Autodesk Inventor part; units mm, degrees
ref_plane "YZ Plane" through (0, 0, 0) normal (1, 0, 0) x (0, 1, 0)
ref_plane "XZ Plane" through (0, 0, 0) normal (0, 1, 0) x (-1, 0, 0)
ref_plane "XY Plane" through (0, 0, 0) normal (0, 0, 1) x (1, 0, 0)
sketch "Sketch1" plane through (0, 0, 0) normal (0, 0, 1) x (1, 0, 0)
  line L0 (24.4, 24.9) -> (-24.4, 24.9)
  line L1 (-24.4, 24.9) -> (-24.4, -24.9)
  line L2 (-24.4, -24.9) -> (24.4, -24.9)
  line L3 (24.4, -24.9) -> (24.4, 24.9)
  circle A0 centre (20.6, 21.8) radius 1.675
  line L4 (0, 24.9) -> (0, -24.9) construction
  line L5 (24.4, 0) -> (-24.4, 0) construction
  circle A1 centre (-20.6, 21.8) radius 1.675
  line L6 (-24.4, 0) -> (24.4, 0) construction
  circle A2 centre (20.6, -21.8) radius 1.675
  circle A3 centre (-20.6, -21.8) radius 1.675
  point P0 (0, 0)
  dimension "d0" = 48.8
  dimension "d1" = 49.8
  dimension "d3" = 3.35
  dimension "d4" = 3.1
  dimension "d5" = 3.8
extrude "Extrusion1" add sketch "Sketch1" along normal blind 2
properties part number "Pomodoro Robot Head's back"
Verification items for the finished model (mm, model axes). Give positions to 0.01 mm unless a question says otherwise; leave off trailing zeros. Order: outer loops, then holes, each group sorted by start corner. A loop starts at its lowest first (then second) coordinate and runs counter-clockwise, first axis right, second up. Notation, with made-up numbers: M -22.5,55.5 L -3.5,55.5 A16 ccw -3.5,68.5 Z; hole C 59,25 d5. An arc over 180 degrees is marked long. Answer in a Markdown table with one row per item. Add a question column.
Item 1: Section check B-B, the plane x = -20.6. Enter the section's corners in (y, z) (3 decimals).
Item 2: Mould release check, pull along Y, two halves, no side actions. Record for faces 1 (the cylindrical face through (-19.827, 23.286, 0.986)), 2 (the flat face through (-24.4, 0, 1)), 3 (the flat face through (0, -24.9, 1)): released by +Y, released by -Y, zero draft, split by the parting line, or undercut.
Item 3: Section check A-A, the plane y = 21.8. Enter the section's corners in (x, z) (3 decimals), and give its area (3 significant figures).
Item 4: Scan lines: probe 1 along Y at (x, z) = (-20.6, 1.4) (3 decimals); probe 2 along Y at (x, z) = (20, 1.3). Record each from-to range of solid material in increasing order. Write a range as from..to.
Filled sheet:
| question | item | result |
|---|---|---|
| 1 | outline | M -24.9,0 L -23.475,0 L -23.475,2 L -24.9,2 Z; M -20.125,0 L 20.125,0 L 20.125,2 L -20.125,2 Z; M 23.475,0 L 24.9,0 L 24.9,2 L 23.475,2 Z |
| 2 | face 1 | undercut |
| 2 | face 2 | zero draft |
| 2 | face 3 | released by -Y |
| 3 | outline | M -24.4,0 L -22.275,0 L -22.275,2 L -24.4,2 Z; M -18.925,0 L 18.925,0 L 18.925,2 L -18.925,2 Z; M 22.275,0 L 24.4,0 L 24.4,2 L 22.275,2 Z |
| 3 | area | 84.2 mm^2 |
| 4 | probe 1 | y = -24.9..-23.475, -20.125..20.125, 23.475..24.9 |
| 4 | probe 2 | y = -24.9..-23.36, -20.24..20.24, 23.36..24.9 |
